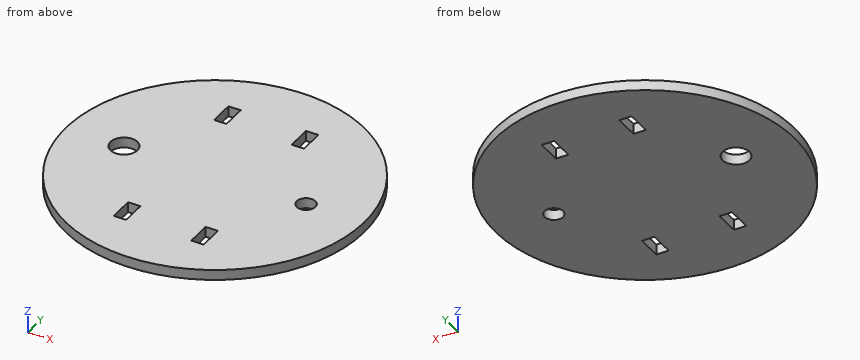
from build123d import *

# Parameters (mm, degrees)
F0_R     = 114.3
F0_W     = 9.525
F0_H     = 19.05
F0_R_2   = 10.31875
F0_R_3   = 7.14375
F1_DEPTH = 7.9375


# Not quite as in the source:
# - a length typed as a fraction of an inch, garbled in the dataset ("3 / 203.2 mm" for 3/8 in), is restored


with BuildPart() as f1:
    # F0 (on Top) → F1 (new body)
    with BuildSketch(Plane.XY):
        Circle(F0_R)
        with Locations((-28.9588448, -66.675)):
            Rectangle(F0_W, F0_H, mode=Mode.SUBTRACT)
        with Locations((30.5463448, -66.675)):
            Rectangle(F0_W, F0_H, mode=Mode.SUBTRACT)
        with Locations((-69.85, 0)):
            Circle(F0_R_2, mode=Mode.SUBTRACT)
        with Locations((-28.9588448, 66.675)):
            Rectangle(F0_W, F0_H, mode=Mode.SUBTRACT)
        with Locations((69.85, 0)):
            Circle(F0_R_3, mode=Mode.SUBTRACT)
        with Locations((30.5463448, 66.675)):
            Rectangle(F0_W, F0_H, mode=Mode.SUBTRACT)
    extrude(amount=F1_DEPTH)


solid = f1.part
Input: part model. Units: mm. Frame: model coordinates. Coordinates: 2 decimals unless noted, no trailing zeros. Loops run counter-clockwise (first coordinate to the right, second up) from the corner with the lowest first, then second, coordinate; pieces in that order, holes last. Notation, with made-up numbers: (15.5, 73.5) -> (53.5, 73.5) arc R14 ccw to (53.5, 83.5) -> close; hole circle Ø1 at (78.25, -34.75). An arc over 180 degrees is marked (long way). One line per item, written item: value.
(1) Ray query, line 1 along X through (y, z) = (-5, 2); line 2 along X through (y, z) = (-2, 6.5); line 3 along Y through (x, z) = (-32, 0.5). Return the intervals inside material, ascending.
Answer below:
line 1: x = -114.19 to -78.88, -60.82 to 64.75, 74.95 to 114.19
line 2: x = -114.28 to -79.97, -59.73 to 62.99, 76.71 to 114.28
line 3: y = -109.73 to -76.2, -57.15 to 57.15, 76.2 to 109.73
(2) Cut plane D-D (x = -69.85). Output: boundary loops of the cut face in (y, z).
Answer below:
outline: (-90.47, 0) -> (-10.32, 0) -> (-10.32, 7.94) -> (-90.47, 7.94) -> close; (10.32, 0) -> (90.47, 0) -> (90.47, 7.94) -> (10.32, 7.94) -> close
(3) Cut plane C-C (x = 69.85). Output: boundary loops of the cut face in (y, z), then the cut area to 3 significant figures.
Answer below:
outline: (-90.47, 0) -> (-7.14, 0) -> (-7.14, 7.94) -> (-90.47, 7.94) -> close; (7.14, 0) -> (90.47, 0) -> (90.47, 7.94) -> (7.14, 7.94) -> close
area: 1,320 mm2
(4) Pin query (flat end, axial travel): pin 1 Ø3 at (x, z) = (-4, 1.5) entering from -Y; pin 2 Ø4 at (x, z) = (28.5, 4) entering from -Y; pin 3 Ø2.5 at (x, z) = (-29.5, 2) entering from -Y. Return the tip coordinate at first contact, or that it passes through.
Answer below:
pin 1: stops at y = -114.27
pin 2: stops at y = -111.19
pin 3: stops at y = -110.75
(5) Cut plane B-B (y = 0). Output: boundary loops of the cut face in (x, z).
Answer below:
outline: (-114.3, 0) -> (-80.17, 0) -> (-80.17, 7.94) -> (-114.3, 7.94) -> close; (-59.53, 0) -> (62.71, 0) -> (62.71, 7.94) -> (-59.53, 7.94) -> close; (76.99, 0) -> (114.3, 0) -> (114.3, 7.94) -> (76.99, 7.94) -> close
(6) Cut plane A-A (z = 5.5). Output: boundary loops of the cut face in (x, y), then the cut area to 3 significant figures.
Answer below:
outline: circle Ø228.6 at (0, 0); hole circle Ø20.64 at (-69.85, 0); hole (-33.72, -76.2) -> (-24.2, -76.2) -> (-24.2, -57.15) -> (-33.72, -57.15) -> close; hole (-33.72, 57.15) -> (-24.2, 57.15) -> (-24.2, 76.2) -> (-33.72, 76.2) -> close; hole (25.78, -76.2) -> (35.31, -76.2) -> (35.31, -57.15) -> (25.78, -57.15) -> close; hole (25.78, 57.15) -> (35.31, 57.15) -> (35.31, 76.2) -> (25.78, 76.2) -> close; hole circle Ø14.29 at (69.85, 0)
area: 39,800 mm2
